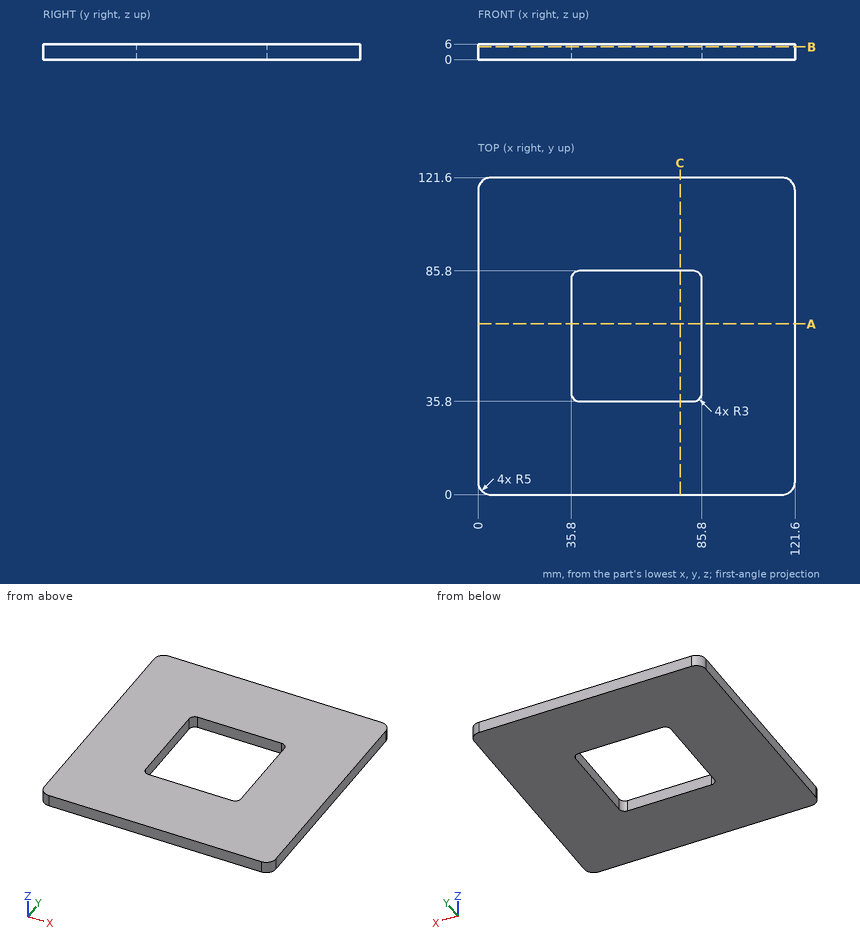
The drawing under review shows one solid part. Ordinate dimensions are in mm from its lowest x, y, z. Give positions to 0.01 mm unless a question says otherwise; leave off trailing zeros. Order: outer loops, then holes, each group sorted by start corner. A loop starts at its lowest first (then second) coordinate and runs counter-clockwise, first axis right, second up. Notation, with made-up numbers: (-11.5, 15) -> (23.5, 15) arc R11 ccw to (23.5, 19) -> close; hole circle Ø9 at (67, -11). An arc over 180 degrees is marked (long way). Write item = value, one per line. Start each with the question number.
(1) To check wall thickness, follow line 1 along Y through (x, z) = (62.5, 2.6); line 2 along Y through (x, z) = (37, 0.75). State the ranges of each line that lie inside material, in increasing order.
(2) We need section B-B on z = 4.9. Write out the cut boundary in (x, y).
(3) We need section A-A on y = 65.5. Write out the cut boundary in (x, z), plus the area to 3 significant figures.
Numbers:
q1.line_1 = 0 to 35.8, 85.8 to 121.6
q1.line_2 = 0 to 36.4, 85.2 to 121.6
q2.outline = (0, 5) arc R5 ccw to (5, 0) -> (116.6, 0) arc R5 ccw to (121.6, 5) -> (121.6, 116.6) arc R5 ccw to (116.6, 121.6) -> (5, 121.6) arc R5 ccw to (0, 116.6) -> close; hole (35.8, 38.8) arc R3 ccw to (38.8, 35.8) -> (82.8, 35.8) arc R3 ccw to (85.8, 38.8) -> (85.8, 82.8) arc R3 ccw to (82.8, 85.8) -> (38.8, 85.8) arc R3 ccw to (35.8, 82.8) -> close
q3.outline = (0, 0) -> (35.8, 0) -> (35.8, 6) -> (0, 6) -> close; (85.8, 0) -> (121.6, 0) -> (121.6, 6) -> (85.8, 6) -> close
q3.area = 430 mm^2
